Work out the finished part from the listing and answer in its coordinate system (mm). Face numbers are marked on the shaded views. Give positions to 0.01 mm unless a question says otherwise; leave off trailing zeros. Order: outer loops, then holes, each group sorted by start corner. A loop starts at its lowest first (then second) coordinate and runs counter-clockwise, first axis right, second up. Notation, with made-up numbers: (-30.5, 75.5) -> (6.5, 75.5) arc R34 cw to (6.5, 107.5) -> close; hole circle Ø3 at (-18.75, -26). An arc over 180 degrees is marked (long way). Answer as CSV lines item,"result". Start each with the question number.
1. A cutting plane is placed at C-C (y = -1.6). Give the vertices of the cut face in (x, z).
2. For a pull along X with two mould halves and no side action, classify the marked faces 1, 2 and 3 as released by +X, released by -X, zero draft, split by the parting line, or undercut.
3. A cutting plane is placed at D-D (x = -2.25). Give the vertices of the cut face in (y, z), then the cut area to 3 significant figures.
4. A cutting plane is placed at B-B (z = 1.25). Give the vertices of the cut face in (x, y), then the cut area to 3 significant figures.
5. Flat-ended cylindrical pins translate along their axes: pin 1 (1 mm diameter, centred on y = -2, z = 7, fed in from +X); pin 2 (2 mm diameter, centred on x = -1, z = 2.5, fed in from -Y); pin 3 (1 mm diameter, centred on x = 0.5, z = 6, fed in from +Y). Find the tip coordinate at first contact, or state that the pin passes through.
6. A cutting plane is placed at A-A (y = -0.8). Give the vertices of the cut face in (x, z), then the cut area to 3 significant figures.
7. Find the intervals of material crossed by L1, parallel to X at y = -0.55, z = 9.5; L2, parallel to X at y = -0.85, z = 10.5; L3, parallel to X at y = -2, z = 1, in increasing order.
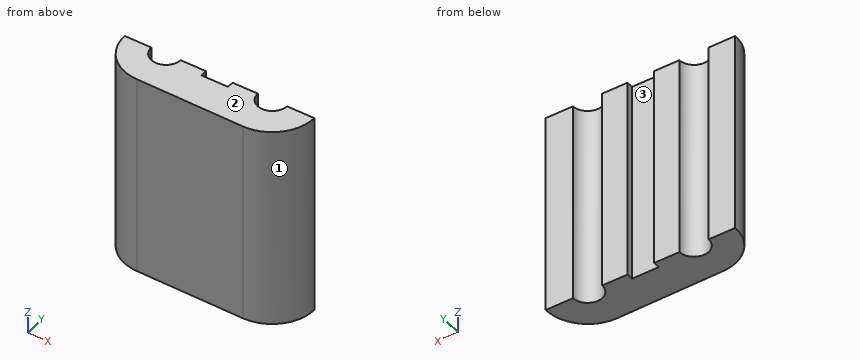
from build123d import *

# Parameters (mm, degrees)
SKETCH1_R           = 1.1
SKETCH1_R_2         = 1.6
BOSS_EXTRUDE1_DEPTH = 15
SKETCH3_R           = 1.6
CUT_EXTRUDE1_DEPTH  = 15
SKETCH5_W           = 2
SKETCH5_H           = 0.5
CUT_EXTRUDE2_DEPTH  = 16


with BuildPart() as part:
    # Sketch1 → Boss-Extrude1 (new body)
    with BuildSketch(Plane.XY):
        with BuildLine():
            Line((-1.61243197, 5.01974999), (-5.34022711, 2.600340269))
            ThreePointArc((-5.34022711, 2.600340269), (-6.625018483, -0.880041239), (-3.652556975, -3.1))
            Line((-3.652556975, -3.1), (4.395993446, -3.201847309))
            ThreePointArc((4.395993446, -3.201847309), (7.362670385, -1.001195929), (6.117333323, 2.476328214))
            Line((6.117333323, 2.476328214), (2.346418367, 4.994010285))
            ThreePointArc((2.346418367, 4.994010285), (0.370849058, 5.59992391), (-1.61243197, 5.01974999))
        make_face()
        with Locations((4.347443025, 0)):
            Circle(SKETCH1_R, mode=Mode.SUBTRACT)
        with Locations((0.347443025, 2)):
            Circle(SKETCH1_R_2, mode=Mode.SUBTRACT)
        with Locations((-3.652556975, 0)):
            Circle(SKETCH1_R, mode=Mode.SUBTRACT)
    extrude(amount=BOSS_EXTRUDE1_DEPTH)

    # Sketch3 → Cut-Extrude1 (cut)
    with BuildSketch(Plane.XY.offset(15)):
        with BuildLine():
            ThreePointArc((-4.752556975, 0), (-3.652556975, 1.1), (-2.552556975, 0))
            Line((-2.552556975, 0), (3.247443025, 0))
            ThreePointArc((3.247443025, 0), (4.347443025, 1.1), (5.447443025, 0))
            Line((5.447443025, 0), (7.49431995, 0))
            ThreePointArc((7.49431995, 0), (7.105300804, 1.404689659), (6.117333323, 2.476328214))
            Line((6.117333323, 2.476328214), (2.346418367, 4.994010285))
            ThreePointArc((2.346418367, 4.994010285), (0.370849058, 5.59992391), (-1.61243197, 5.01974999))
            Line((-1.61243197, 5.01974999), (-5.34022711, 2.600340269))
            ThreePointArc((-5.34022711, 2.600340269), (-6.376687792, 1.479564561), (-6.752556975, 0))
            Line((-6.752556975, 0), (-4.752556975, 0))
        make_face()
        with Locations((0.347443025, 2)):
            Circle(SKETCH3_R, mode=Mode.SUBTRACT)
    extrude(amount=-CUT_EXTRUDE1_DEPTH, mode=Mode.SUBTRACT)

    # Sketch5 → Cut-Extrude2 (cut, through all)
    with BuildSketch(Plane.XY.offset(15)):
        with Locations((0.347443025, -0.25)):
            Rectangle(SKETCH5_W, SKETCH5_H)
    extrude(amount=-CUT_EXTRUDE2_DEPTH, mode=Mode.SUBTRACT)


solid = part.part
Answer sheet:
1,outline,"(-6.31, 0) -> (7.11, 0) -> (7.11, 15) -> (-6.31, 15) -> close"
2,face 1,"released by +X"
2,face 2,"zero draft"
2,face 3,"undercut"
3,outline,"(-3.12, 0) -> (0, 0) -> (0, 15) -> (-3.12, 15) -> close"
3,area,"46.8 mm^2"
4,outline,"(-6.75, 0) arc R3.1 ccw to (-3.65, -3.1) -> (4.4, -3.2) arc R3.1 ccw to (7.49, 0) -> (5.45, 0) arc R1.1 cw to (3.25, 0) -> (1.35, 0) -> (1.35, -0.5) -> (-0.65, -0.5) -> (-0.65, 0) -> (-2.55, 0) arc R1.1 cw to (-4.75, 0) -> close"
4,area,"36.0 mm^2"
5,pin 1,"stops at x = 7.16"
5,pin 2,"stops at y = -3.15"
5,pin 3,"stops at y = -0.5"
6,outline,"(-6.65, 0) -> (-4.41, 0) -> (-4.41, 15) -> (-6.65, 15) -> close; (-2.9, 0) -> (3.59, 0) -> (3.59, 15) -> (-2.9, 15) -> close; (5.1, 0) -> (7.42, 0) -> (7.42, 15) -> (5.1, 15) -> close"
6,area,"166 mm^2"
7,L1,"x = -6.7 to -4.61, -2.7 to 3.39, 5.3 to 7.46"
7,L2,"x = -6.63 to -4.35, -2.95 to 3.65, 5.05 to 7.4"
7,L3,"x = -6.02 to 6.85"
